Read the model definition and answer for the solid it produces. Units are mm, in the model's axes. Face numbers are marked on the shaded views. A direction names the side the tool comes from. Round coordinates to 2 decimals unless told otherwise and drop trailing zeros. Order: outer loops, then holes, each group sorted by start corner. A loop starts at its lowest first (then second) coordinate and runs counter-clockwise, first axis right, second up.
from build123d import *

# Parameters (mm, degrees)
F2_W     = 0.508
F2_H     = 0.508
F3_DEPTH = 3.81


# Not quite as in the source:
# - a pattern or mirror of a feature is missing from the dataset's text; its kind, count and spacing are read off the source's solid


with BuildPart() as f1:
    # F0 (on Front) → F1 (revolve)
    with BuildSketch(Plane.XZ):
        with BuildLine():
            Line((0, 4.5974), (0, 0))
            Line((0, 0), (1.6002, 0))
            Line((1.6002, 0), (1.6002, 0.9906))
            Line((1.6002, 0.9906), (1.397, 0.9906))
            Line((1.397, 0.9906), (1.397, 3.2004))
            ThreePointArc((1.397, 3.2004), (0.9878281733, 4.1882281733), (0, 4.5974))
        make_face()
    revolve(axis=Axis((0, 0, 2.2987), (0, 0, 1)))

    # F2 (on face) → F3 (join)
    with BuildSketch(Plane(origin=(0, 0, 0), x_dir=(1, 0, 0), z_dir=(0, 0, -1))):
        with Locations((1.27, 0)):
            Rectangle(F2_W, F2_H)
    f3 = extrude(amount=F3_DEPTH)

    # F3_copies: F3 across plane
    add(f3.mirror(Plane(origin=(0, 0, 0), x_dir=(0, 0, -1), z_dir=(-1, 0, 0))))


solid = f1.part
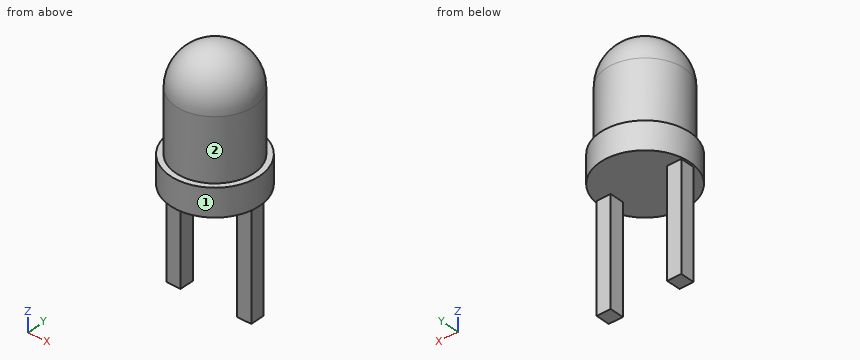
Q1. Flat-ended cylindrical pins translate along their axes: pin 1 (0.6 mm diameter, centred on y = 0, z = -1, fed in from -X); pin 2 (0.6 mm diameter, centred on y = 0, z = -1.5, fed in from +X); pin 3 (0.6 mm diameter, centred on x = -1.5, z = -1.5, fed in from -Y). Find the tip coordinate at first contact, or state that the pin passes through.
Outcome:
pin 1: stops at x = -1.52
pin 2: stops at x = 1.52
pin 3: stops at y = -0.25
Q2. For the marked faces 1 and 2, determine the directions among +Z, -Z, +X, -X, +Y, -Y from which every point of the face is accessible in a straight line to the end or side of a thin tool.
Outcome:
face 1: +Z, -Z
face 2: +Z
Q3. A cutting plane is placed at C-C, the plane x = 0. Give the vertices of the cut face in (y, z), plus the area to 3 significant figures.
Outcome:
outline: (-1.6, 0) - (1.6, 0) - (1.6, 0.99) - (1.4, 0.99) - (1.4, 3.2) arc R1.4 ccw to (-1.4, 3.2) - (-1.4, 0.99) - (-1.6, 0.99) - close
area: 12.4 mm2
Q4. Straight lines are drawn through the part: probe 1 along X at (y, z) = (0.15, -0.25); probe 2 along Y at (x, z) = (1.35, -1.75); probe 3 along Z at (x, y) = (-1.05, 1). For each, find the intervals that lie inside material, in ascending order.
Outcome:
probe 1: x = -1.52 to -1.02, 1.02 to 1.52
probe 2: y = -0.25 to 0.25
probe 3: z = 0 to 0.99
Q5. A cutting plane is placed at B-B, the plane z = -3. Give the vertices of the cut face in (x, y), plus the area to 3 significant figures.
Outcome:
outline: (-1.52, -0.25) - (-1.02, -0.25) - (-1.02, 0.25) - (-1.52, 0.25) - close; (1.02, -0.25) - (1.52, -0.25) - (1.52, 0.25) - (1.02, 0.25) - close
area: 0.516 mm2
Q6. A cutting plane is placed at D-D, the plane z = 0.5. Give the vertices of the cut face in (x, y).
Outcome:
outline: circle Ø3.2 at (0, 0)
Q7. A cutting plane is placed at A-A, the plane y = 0. Give the vertices of the cut face in (x, z), plus the area to 3 significant figures.
Outcome:
outline: (-1.6, 0) - (-1.52, 0) - (-1.52, -3.81) - (-1.02, -3.81) - (-1.02, 0) - (1.02, 0) - (1.02, -3.81) - (1.52, -3.81) - (1.52, 0) - (1.6, 0) - (1.6, 0.99) - (1.4, 0.99) - (1.4, 3.2) arc R1.4 ccw to (-1.4, 3.2) - (-1.4, 0.99) - (-1.6, 0.99) - close
area: 16.3 mm2
